The model under review builds one solid part; all positions refer to its coordinate system, in mm. Give positions to 0.01 mm unless a question says otherwise; leave off trailing zeros. Loops run counter-clockwise (first coordinate to the right, second up) from the corner with the lowest first, then second, coordinate; pieces in that order, holes last. Notation, with made-up numbers: M 9.5,54.25 L 21.5,54.25 A20 cw 21.5,90.25 Z; hole C -7.75,41.25 d11. An arc over 180 degrees is marked long. Return JSON: item names as keys, results as strings.
Autodesk Inventor part; units mm, degrees
ref_plane "YZ Plane" through (0, 0, 0) normal (1, 0, 0) x (0, 1, 0)
ref_plane "XZ Plane" through (0, 0, 0) normal (0, 1, 0) x (-1, 0, 0)
ref_plane "XY Plane" through (0, 0, 0) normal (0, 0, 1) x (1, 0, 0)
sketch "Sketch1" plane through (0, 0, 0) normal (0, 0, 1) x (1, 0, 0)
  line L0 (0, 0) -> (50.8, 0)
  line L1 (50.8, 0) -> (50.8, 169.8752)
  line L2 (50.8, 169.8752) -> (0, 169.8752)
  line L3 (0, 169.8752) -> (0, 0)
  line L4 (25.4, 169.8752) -> (25.4, 144.4752)
  line L5 (25.4, 169.8752) -> (50.8, 169.8752) construction
  circle A0 centre (25.4, 144.4752) radius 14.2875
  line L6 (25.4, 144.4752) -> (43.3605, 162.4357)
  line L7 (25.4, 144.4752) -> (50.8, 144.4752) construction
  line L8 (7.4395, 126.5147) -> (43.3605, 126.5147)
  line L9 (43.3605, 162.4357) -> (7.4395, 162.4357)
  line L10 (7.4395, 162.4357) -> (7.4395, 126.5147)
  circle A1 centre (7.4395, 162.4357) radius 2.032
  circle A2 centre (7.4395, 126.5147) radius 2.032
  circle A3 centre (43.3605, 162.4357) radius 2.032
  circle A4 centre (43.3605, 126.5147) radius 2.032
  line L11 (0, 0) -> (50.8, 0)
  line L12 (50.8, 0) -> (50.8, 38.1)
  line L13 (0, 38.1) -> (0, 0)
  line L14 (25.4, 38.1) -> (12.7, 38.1)
  line L15 (25.4, 38.1) -> (38.1, 38.1) construction
  line L16 (12.7, 38.1) -> (38.1, 38.1)
  circle A5 centre (12.7, 38.1) radius 3.175
  circle A6 centre (38.1, 38.1) radius 3.175
  dimension "d0" = 50.8
  dimension "d1" = 169.8752
  dimension "d2" = 25.4
  dimension "d3" = 90
  dimension "d4" = 28.575
  dimension "d5" = 25.4
  dimension "d6" = 45
  dimension "d7" = 50.8
  dimension "d9" = 4.064
  dimension "d10" = 4.064
  dimension "d11" = 4.064
  dimension "d12" = 4.064
  dimension "d13" = 50.8
  dimension "d14" = 38.1
  dimension "d15" = 12.7
  dimension "d16" = 180
  dimension "d17" = 25.4
  dimension "d18" = 0
  dimension "d19" = 6.35
  dimension "d20" = 6.35
extrude "Extrusion1" add sketch "Sketch1" along normal blind 25.4 contours L9 A3 L6 A0 L4 | L3 L2 L1 L0
sketch "Sketch2" plane through (0, 169.8752, 0) normal (0, 1, 0) x (1, 0, 0)
  line L0 (0, 0) -> (3.175, 0)
  line L1 (3.175, 0) -> (3.175, -3.175)
  line L2 (3.175, -3.175) -> (0, -3.175)
  line L3 (0, -3.175) -> (0, 0)
  line L4 (3.175, -3.175) -> (47.625, -3.175)
  line L5 (47.625, -3.175) -> (47.625, -22.225)
  line L6 (47.625, -22.225) -> (3.175, -22.225)
  line L7 (3.175, -22.225) -> (3.175, -3.175)
  dimension "d23" = 3.175
  dimension "d24" = 3.175
  dimension "d25" = 44.45
  dimension "d26" = 19.05
extrude "Extrusion2" cut sketch "Sketch2" against normal blind 254 contours L4 L5 L6 L7
sketch "Sketch3" plane through (0, 0, 25.4) normal (0, 0, 1) x (1, 0, 0)
  circle A0 centre (12.7, 38.1) radius 3.175
  line L0 (12.7, 38.1) -> (38.1, 38.1)
  line L1 (38.1, 38.1) -> (38.1, 12.7)
  line L2 (38.1, 12.7) -> (12.7, 12.7)
  line L3 (12.7, 12.7) -> (12.7, 38.1)
  circle A1 centre (12.7, 12.7) radius 3.175
  circle A2 centre (38.1, 12.7) radius 3.175
  dimension "d29" = 25.4
  dimension "d30" = 25.4
  dimension "d31" = 6.35
  dimension "d32" = 6.35
extrude "Extrusion3" cut sketch "Sketch3" against normal blind 25.4 contours A1 L2 L3 | L3 L2 A1 | A2 L2 L1 | L1 L2 A2
sketch "Sketch4" plane through (0, 169.8752, 0) normal (0, 1, 0) x (1, 0, 0)
  line L0 (47.625, -22.225) -> (3.175, -22.225)
  line L1 (3.175, -22.225) -> (3.175, -3.175)
  line L2 (3.175, -3.175) -> (47.625, -3.175)
  line L3 (47.625, -3.175) -> (47.625, -22.225)
  line L4 (50.8, 0) -> (50.8, -25.4)
  line L5 (0, 0) -> (50.8, 0)
  line L6 (50.8, 0) -> (50.8, -22.225)
  line L7 (50.8, -22.225) -> (0, -22.225)
  line L8 (0, -22.225) -> (0, 0)
extrude "Extrusion4" cut sketch "Sketch4" against normal blind 254 contours L3 L2 L1 L7 L8 L5 L4
sketch "Sketch5" plane through (0, 0, 25.4) normal (0, 0, 1) x (1, 0, 0)
  circle A0 centre (38.1, 12.7) radius 3.175
  circle A1 centre (12.7, 12.7) radius 3.175
  circle A2 centre (25.4, 144.4752) radius 14.2875
  circle A3 centre (38.1, 38.1) radius 3.175
  circle A4 centre (12.7, 38.1) radius 3.175
  circle A5 centre (43.3605, 126.5147) radius 2.032
  circle A6 centre (43.3605, 162.4357) radius 2.032
  circle A7 centre (7.4395, 126.5147) radius 2.032
  circle A8 centre (7.4395, 162.4357) radius 2.032
  line L0 (0, 0) -> (50.8, 0)
  line L1 (50.8, 0) -> (50.8, 169.8752)
  line L2 (50.8, 169.8752) -> (0, 169.8752)
  line L3 (0, 169.8752) -> (0, 0)
extrude "Extrusion5" add sketch "Sketch5" along normal blind 3.175
sketch "Sketch6" plane through (0, 0, 28.575) normal (0, 0, 1) x (1, 0, 0)
  circle A0 centre (25.4, 144.4752) radius 14.2875
  circle A1 centre (25.4, 144.4752) radius 9.525
  dimension "d39" = 19.05
extrude "Extrusion6" add sketch "Sketch6" against normal blind 6.35
sketch "Sketch7" plane through (0, 0, 28.575) normal (0, 0, 1) x (1, 0, 0)
  line L0 (50.8, 169.8752) -> (0, 169.8752)
  line L1 (0, 169.8752) -> (0, 0)
  line L2 (25.4, 169.8752) -> (25.4, 95.25)
  line L3 (25.4, 169.8752) -> (100.0252, 169.8752) construction
  circle A0 centre (25.4, 95.25) radius 7.9375
  dimension "d43" = 74.6252
  dimension "d44" = 90
  dimension "d45" = 15.875
extrude "Extrusion7" cut sketch "Sketch7" against normal blind 25.4
sketch "Sketch8" plane through (0, 0, 28.575) normal (0, 0, 1) x (1, 0, 0)
  circle A0 centre (25.4, 144.4752) radius 9.525
  circle A1 centre (25.4, 144.4752) radius 14.2875
  dimension "d48" = 28.575
extrude "Extrusion8" cut sketch "Sketch8" against normal blind 25.4
sketch "Sketch9" plane through (0, 0, 28.575) normal (0, 0, 1) x (1, 0, 0)
  circle A0 centre (25.4, 95.25) radius 7.9375
  circle A1 centre (7.4395, 162.4357) radius 2.032
  circle A2 centre (7.4395, 126.5147) radius 2.032
  circle A3 centre (43.3605, 162.4357) radius 2.032
  circle A4 centre (43.3605, 126.5147) radius 2.032
  line L0 (25.4, 95.25) -> (43.3605, 113.2105)
  line L1 (25.4, 95.25) -> (50.8, 95.25) construction
  line L2 (43.3605, 113.2105) -> (7.4395, 77.2895)
  circle A5 centre (7.4395, 113.2105) radius 2.032
  circle A6 centre (43.3605, 113.2105) radius 2.032
  circle A7 centre (43.3605, 77.2895) radius 2.032
  circle A8 centre (7.4395, 77.2895) radius 2.032
  dimension "d51" = 25.4
  dimension "d52" = 45
  dimension "d53" = 50.8
  dimension "d54" = 0
  dimension "d55" = 4.064
  dimension "d56" = 4.064
  dimension "d57" = 4.064
  dimension "d58" = 4.064
extrude "Extrusion9" cut sketch "Sketch9" against normal blind 6.35 contours A8 | A6 | A1 | A2 | A3 | A4 | A5 | A7
sketch "Sketch10" plane through (0, 0, 28.575) normal (0, 0, 1) x (1, 0, 0)
  circle A0 centre (7.4395, 162.4357) radius 2.032
  circle A1 centre (7.4395, 126.5147) radius 2.032
  circle A2 centre (43.3605, 162.4357) radius 2.032
  circle A3 centre (43.3605, 126.5147) radius 2.032
extrude "Extrusion10" add sketch "Sketch10" against normal blind 6.35
sketch "Sketch11" plane through (0, 0, 28.575) normal (0, 0, 1) x (1, 0, 0)
  circle A0 centre (25.4, 144.4752) radius 14.2875
  line L0 (0, 169.8752) -> (50.8, 169.8752)
  line L1 (50.8, 169.8752) -> (50.8, 119.0752)
  line L2 (50.8, 119.0752) -> (0, 119.0752)
  line L3 (0, 119.0752) -> (0, 169.8752)
  dimension "d64" = 50.8
  dimension "d65" = 50.8
extrude "Extrusion11" cut sketch "Sketch11" against normal blind 25.4
sketch "Sketch12" plane through (0, 0, 28.575) normal (0, 0, 1) x (1, 0, 0)
  line L0 (50.8, 0) -> (50.8, 119.0752)
  circle A0 centre (25.4, 95.25) radius 7.9375
  line L1 (25.4, 95.25) -> (25.4, 139.7)
  line L2 (25.4, 95.25) -> (69.85, 95.25) construction
  circle A1 centre (25.4, 139.7) radius 14.2875
  line L3 (25.4, 139.7) -> (25.4, 165.1)
  line L4 (25.4, 139.7) -> (50.8, 139.7) construction
  line L5 (25.4, 165.1) -> (0, 165.1)
  line L6 (0, 165.1) -> (50.8, 165.1)
  line L7 (50.8, 165.1) -> (50.8, 119.0752)
  line L8 (50.8, 119.0752) -> (0, 119.0752)
  line L9 (0, 119.0752) -> (0, 165.1)
  dimension "d68" = 44.45
  dimension "d69" = 90
  dimension "d70" = 28.575
  dimension "d71" = 25.4
  dimension "d72" = 90
  dimension "d73" = 25.4
  dimension "d74" = 90
extrude "Extrusion12" add sketch "Sketch12" against normal blind 6.35 contours L8 L9 L5 L3 A1 L1 | L1 A1 L3 L6 L7 L8
properties part number "Z-Plate-Gears"
1) Consider section C-C on y = 38.1. Write out the cut boundary in (x, z) (3 decimals).
From the geometry:
{"outline": "M 0,22.225 L 9.525,22.225 L 9.525,28.575 L 0,28.575 Z; M 15.875,22.225 L 34.925,22.225 L 34.925,28.575 L 15.875,28.575 Z; M 41.275,22.225 L 50.8,22.225 L 50.8,28.575 L 41.275,28.575 Z"}
2) Consider section B-B on x = 25.4. Write out the cut boundary in (y, z) (1 decimal), then the cut area to 3 significant figures.
From the geometry:
{"outline": "M 0,22.2 L 87.3,22.2 L 87.3,28.6 L 0,28.6 Z; M 103.2,22.2 L 125.4,22.2 L 125.4,28.6 L 103.2,28.6 Z; M 154,22.2 L 165.1,22.2 L 165.1,28.6 L 154,28.6 Z", "area": "766 mm²"}
3) Wall thickness on L1, parallel to Y at x = 25.4, z = 25.25; L2, parallel to X at y = 77.5, z = 23; L3, parallel to X at y = 38.1, z = 24 (3 decimals): over which ranges is each line inside the solid? List them lowest first. Write a range as from..to.
From the geometry:
{"L1": "0..87.31, 103.19..125.41, 153.99..165.1", "L2": "0..5.42, 9.46..41.34, 45.38..50.8", "L3": "0..9.525, 15.875..34.925, 41.275..50.8"}
4) The part is to be moulded in two halves that separate along X. For faces 1 (the face through (50.8, 81, 25)), 2 (the face through (25, 84, 28.575)), 3 (the face through (10.18, 10.77, 25.44)), 4 (the face through (23.54, 153.866, 25.444)), say which applies: released by +X, released by -X, zero draft, split by the parting line, or undercut.
From the geometry:
{"face 1": "released by +X", "face 2": "zero draft", "face 3": "undercut", "face 4": "undercut"}
5) Consider section A-A on y = 139.7. Write out the cut boundary in (x, z) (1 decimal).
From the geometry:
{"outline": "M 0,22.2 L 11.1,22.2 L 11.1,28.6 L 0,28.6 Z; M 39.7,22.2 L 50.8,22.2 L 50.8,28.6 L 39.7,28.6 Z"}
6) Consider section D-D on x = 38.1. Write out the cut boundary in (y, z) (3 decimals).
From the geometry:
{"outline": "M 0,22.225 L 9.525,22.225 L 9.525,28.575 L 0,28.575 Z; M 15.875,22.225 L 34.925,22.225 L 34.925,28.575 L 15.875,28.575 Z; M 41.275,22.225 L 133.155,22.225 L 133.155,28.575 L 41.275,28.575 Z; M 146.245,22.225 L 165.1,22.225 L 165.1,28.575 L 146.245,28.575 Z"}
